from build123d import *

# Parameters (mm, degrees)
BOSS_EXTRUDE1_START = -88.9
BOSS_EXTRUDE1_DEPTH = 393.7
SKETCH3_R           = 2.4892
CUT_EXTRUDE2_DEPTH  = 51.8


with BuildPart() as part:
    # Sketch1 → Boss-Extrude1 (new body)
    with BuildSketch(Plane(origin=(0, 0, 0), x_dir=(-1, 0, 0), z_dir=(0, 0, -1)).offset(BOSS_EXTRUDE1_START)):
        with BuildLine():
            Line((-12.7, 25.146), (-12.7, -25.146))
            ThreePointArc((-12.7, -25.146), (-12.625605122, -25.325605122), (-12.446, -25.4))
            Line((-12.446, -25.4), (12.446, -25.4))
            ThreePointArc((12.446, -25.4), (12.625605122, -25.325605122), (12.7, -25.146))
            Line((12.7, -25.146), (12.7, 25.146))
            ThreePointArc((12.7, 25.146), (12.625605122, 25.325605122), (12.446, 25.4))
            Line((12.446, 25.4), (-12.446, 25.4))
            ThreePointArc((-12.446, 25.4), (-12.625605122, 25.325605122), (-12.7, 25.146))
        make_face()
        with BuildLine():
            Line((-11.1125, -22.225), (-11.1125, 22.225))
            ThreePointArc((-11.1125, 22.225), (-10.647532015, 23.347532015), (-9.525, 23.8125))
            Line((-9.525, 23.8125), (9.525, 23.8125))
            ThreePointArc((9.525, 23.8125), (10.647532015, 23.347532015), (11.1125, 22.225))
            Line((11.1125, 22.225), (11.1125, -22.225))
            ThreePointArc((11.1125, -22.225), (10.647532015, -23.347532015), (9.525, -23.8125))
            Line((9.525, -23.8125), (-9.525, -23.8125))
            ThreePointArc((-9.525, -23.8125), (-10.647532015, -23.347532015), (-11.1125, -22.225))
        make_face(mode=Mode.SUBTRACT)
    extrude(amount=-BOSS_EXTRUDE1_DEPTH)

    # Sketch3 → Cut-Extrude2 (cut, through all)
    with BuildSketch(Plane.XZ.offset(25.4)):
        with Locations((0, 165.1)):
            Circle(SKETCH3_R)
        with Locations((0, 190.5)):
            Circle(SKETCH3_R)
        with Locations((0, 215.9)):
            Circle(SKETCH3_R)
        with Locations((0, 241.3)):
            Circle(SKETCH3_R)
        with Locations((0, 266.7)):
            Circle(SKETCH3_R)
        with Locations((0, 292.1)):
            Circle(SKETCH3_R)
        with Locations((0, 317.5)):
            Circle(SKETCH3_R)
        with Locations((0, 342.9)):
            Circle(SKETCH3_R)
        with Locations((0, 368.3)):
            Circle(SKETCH3_R)
        with Locations((0, 393.7)):
            Circle(SKETCH3_R)
        with Locations((0, 419.1)):
            Circle(SKETCH3_R)
        with Locations((0, 444.5)):
            Circle(SKETCH3_R)
    extrude(amount=-CUT_EXTRUDE2_DEPTH, mode=Mode.SUBTRACT)


solid = part.part
Check sheet for the modelled part. Datum: model origin and axes. Units: mm. A direction names the side the tool comes from. Give positions to 0.01 mm unless a question says otherwise; leave off trailing zeros. Order: outer loops, then holes, each group sorted by start corner. A loop starts at its lowest first (then second) coordinate and runs counter-clockwise, first axis right, second up. Notation, with made-up numbers: M 5,11 L 37,11 A15 ccw 37,16 Z; hole C -29,21 d4. An arc over 180 degrees is marked long. Answer as CSV lines item,"result". Start each with the question number.
Item 1: Tool access check on faces 1 (the face through (11.3, 2, 88.9)), 2 (the face through (0, -23.812, 283)). Record the directions out of +Z, -Z, +X, -X, +Y, -Y that give a thin tool (end or side, any length) a straight path to the whole face; none if there is none.
Item 2: Thickness scan on line 1 (X direction, y = 6, z = 231); line 2 (X direction, y = -24.3, z = 266.7); line 3 (Y direction, x = 8.25, z = 314). Record the ranges inside material, lowest first. Write a range as [from, to].
Item 3: Gauge pin test, flat end, axial feed: P1, Ø8, axis at x = 0, z = 342.9, coming from the +Y side. Record the tip position at first contact, or that the pin passes through.
Item 4: Cross-section at A-A on y = 8. Enter the section's corners in (x, z).
Item 5: Mould release check, pull along X, two halves, no side actions. Record for faces 3 (the face through (-11.112, 0, 283)), 4 (the face through (11.112, 0, 283)), 5 (the face through (11.3, 2, 482.6)), 6 (the face through (12.7, 0, 283)): +X half, -X half, draft (parallel to the pull), parting line (faces both ways), or undercut.
Established:
1,face 1,"-Z, +X, -X, +Y, -Y"
1,face 2,"+Z, -Z"
2,line 1,"x = [-12.7, -11.11], [11.11, 12.7]"
2,line 2,"x = [-12.7, -2.49], [2.49, 12.7]"
2,line 3,"y = [-25.4, -23.81], [23.81, 25.4]"
3,P1,"stops at y = 25.4"
4,outline,"M -12.7,88.9 L -11.11,88.9 L -11.11,482.6 L -12.7,482.6 Z; M 11.11,88.9 L 12.7,88.9 L 12.7,482.6 L 11.11,482.6 Z"
5,face 3,"undercut"
5,face 4,"undercut"
5,face 5,"draft"
5,face 6,"+X half"
